```python
from build123d import *

# Parameters (mm, degrees)
F1_DEPTH = 4572
F2_SCALE = 0.0393700787
F3_ANGLE = 180


with BuildPart() as f1:
    # F0 (on Top) → F1 (new body)
    with BuildSketch(Plane.XY):
        Polygon((508, 0), (0, 0), (-508, 0), (-508, 762), (-1270, 762), (-1270, 0), (-2286, 0), (-2286, -457.2), (0, -457.2), (2286, -457.2), (2286, 0), (1270, 0), (1270, 762), (508, 762), align=None)
    extrude(amount=F1_DEPTH)


with BuildPart() as f1_1:
    # F2: moved
    add(f1.part.scale(F2_SCALE))


with BuildPart() as f1_2:
    # F3: moved
    add(f1_1.part.rotate(Axis((0, 0, 0), (1, 0, 0)), F3_ANGLE))


solid = f1_2.part
```
Could you check a few things on this model? Use its own coordinates, in mm. A direction names the side the tool comes from. Round coordinates to 2 decimals unless told otherwise and drop trailing zeros. Loops run counter-clockwise (first coordinate to the right, second up) from the corner with the lowest first, then second, coordinate; pieces in that order, holes last.
Q1. Please list where these lines run through material, in increasing order: L1, parallel to X at y = -27, z = -8; L2, parallel to Y at x = -70.5, z = -67.5.
Q2. On a 3-axis mill with a long thin cutter (end or side, diameter ignored), from which of +Z, -Z, +X, -X, +Y, -Y can I reach the whole of each face in a straight line? I mean faces 4 (the flat face through (70, 0, -89)), 5 (the flat face through (-50, -15, -89)), 6 (the flat face through (0, 0, -89)). Say none if no direction works.
Q3. I want a section at B-B (z = -75). Write out the boundary of the cut face in (x, y).
Q4. I want a section at C-C (x = 5). Write out the boundary of the cut face in (y, z), and give its area (3 significant figures).
Q5. For P1, Ø8, axis at y = -3.5, z = -144, coming from the +X side; P2, Ø15, axis at y = -11.5, z = -61, coming from the -X side; P3, Ø15, axis at y = -11.5, z = -72.5, coming from the +X side; P4, Ø12, axis at x = 70, z = -103.5, coming from the -Y side, each with a flat end and sliding along its axis, tell me the tip position at first contact or that it passes through.
Q6. I want a section at A-A (y = -11.5). Write out the boundary of the cut face in (x, z).
Q7. Thinking about a two-plate mould opening in X: for faces 1 (the flat face through (50, -15, -89)), 2 (the flat face through (20, -15, -89)), 3 (the flat face through (-1, 4, -180)), which applies, pulls with the +X half, pulls with the -X half, needs draft (parallel to the pull), parting line crosses it, or undercut?
Answer below:
1. L1: x = -50 to -20, 20 to 50
1. L2: y = 0 to 18
2. face 4: +Z, -Z, +X, -Y
2. face 5: +Z, -Z, -X, -Y
2. face 6: +Z, -Z, -Y
3. outline: (-90, 0) - (-50, 0) - (-50, -30) - (-20, -30) - (-20, 0) - (20, 0) - (20, -30) - (50, -30) - (50, 0) - (90, 0) - (90, 18) - (-90, 18) - close
4. outline: (0, -180) - (18, -180) - (18, 0) - (0, 0) - close
4. area: 3,240 mm2
5. P1: stops at x = 90
5. P2: stops at x = -50
5. P3: stops at x = 50
5. P4: stops at y = 0
6. outline: (-50, -180) - (-20, -180) - (-20, 0) - (-50, 0) - close; (20, -180) - (50, -180) - (50, 0) - (20, 0) - close
7. face 1: pulls with the +X half
7. face 2: undercut
7. face 3: needs draft
